Read the model definition and answer for the solid it produces. Units are mm, in the model's axes. A direction names the side the tool comes from. Coordinates: 2 decimals unless noted, no trailing zeros. Order: outer loops, then holes, each group sorted by start corner. A loop starts at its lowest first (then second) coordinate and runs counter-clockwise, first axis right, second up. Notation, with made-up numbers: (4.5, 22) - (41.5, 22) arc R28 cw to (41.5, 42) - close; hole circle Ø1 at (67.25, -26). An arc over 180 degrees is marked (long way). Use one line per item in the form item = value.
```python
from build123d import *

# Parameters (mm, degrees)
SKETCH1_W           = 19.5
SKETCH1_H           = 21.5
BOSS_EXTRUDE1_DEPTH = 0.508
SKETCH2_R           = 5.08
BOSS_EXTRUDE2_DEPTH = 5.08
FILLET1_R           = 1.27


with BuildPart() as part:
    # Sketch1 → Boss-Extrude1 (new body)
    with BuildSketch(Plane(origin=(0, 0, 0), x_dir=(1, 0, 0), z_dir=(0, 1, 0))):
        Rectangle(SKETCH1_W, SKETCH1_H)
    extrude(amount=BOSS_EXTRUDE1_DEPTH)

    # Sketch2 → Boss-Extrude2 (add)
    with BuildSketch(Plane(origin=(0, 0, 0), x_dir=(1, 0, 0), z_dir=(0, 1, 0))):
        Circle(SKETCH2_R)
    extrude(amount=BOSS_EXTRUDE2_DEPTH)

    # Fillet1
    fillet1_edges = [part.edges().sort_by_distance(p)[0] for p in [
        (-5.08, 0.508, 0),
        (-5.08, 5.08, 0),
    ]]
    fillet(fillet1_edges, radius=FILLET1_R)


solid = part.part
```
(1) Which of the six approach directions +Z, -Z, +X, -X, +Y, -Y give full straight-line access (tool end or side, diameter ignored) to faces 1 (the flat face through (0, 5.08, 0)), 2 (the cylindrical face through (-0.661, 2.78, -5.037))?
Answer list:
face_1 = +Z, -Z, +X, -X, +Y
face_2 = +Y
(2) Section B-B, the plane y = 2.8 is taken. Write down the section's boundary in (x, z), then the cut area to 3 significant figures.
Answer list:
outline = circle Ø10.16 at (0, 0)
area = 81.1 mm2
(3) Section C-C, the plane z = 9.5 is taken. Write down the section's boundary in (x, y), then the cut area to 3 significant figures.
Answer list:
outline = (-9.75, 0) - (9.75, 0) - (9.75, 0.51) - (-9.75, 0.51) - close
area = 9.91 mm2
(4) Given pin 1 Ø1 at (x, z) = (-5.5, -5.5) entering from -Y; pin 2 Ø3 at (y, z) = (3.5, 5) entering from -X, each flat-ended and moving along its own axis, determine where each tip first touches the part or whether it passes through.
Answer list:
pin_1 = 0
pin_2 = -3.68
(5) Section A-A, the plane z = 0 is taken. Write down the section's boundary in (x, y).
Answer list:
outline = (-9.75, 0) - (9.75, 0) - (9.75, 0.51) - (6.35, 0.51) arc R1.27 cw to (5.08, 1.78) - (5.08, 3.81) arc R1.27 ccw to (3.81, 5.08) - (-3.81, 5.08) arc R1.27 ccw to (-5.08, 3.81) - (-5.08, 1.78) arc R1.27 cw to (-6.35, 0.51) - (-9.75, 0.51) - close
(6) Straight lines are drawn through the part: L1, parallel to Y at x = 8, z = 10; L2, parallel to Z at x = 0.25, y = 3.45; L3, parallel to Z at x = 4.75, y = 1.05. For each, find the intervals that lie inside material, in ascending order.
Answer list:
L1 = 0 to 0.51
L2 = -5.07 to 5.07
L3 = -2.37 to 2.37
